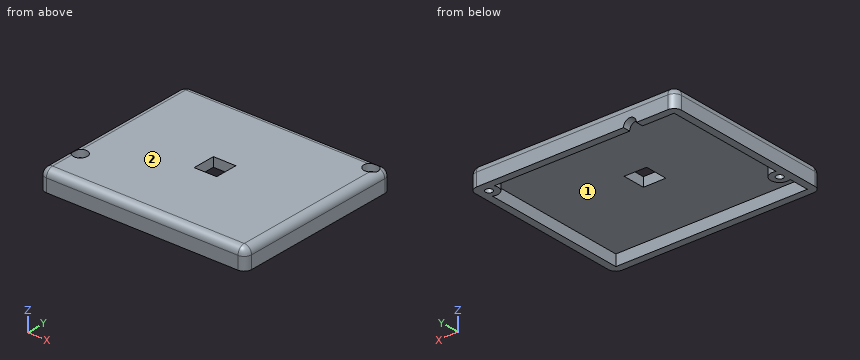
Autodesk Inventor part; units mm, degrees
ref_plane "Arbeitsebene1" through (26, 12.1004, 0) normal (0, 0, 1) x (1, 0, 0)
ref_plane "YZ Plane" through (0, 0, 0) normal (1, 0, 0) x (0, 1, 0)
ref_plane "XZ Plane" through (0, 0, 0) normal (0, 1, 0) x (-1, 0, 0)
ref_plane "Arbeitsebene1" through (26, 12.1004, 0) normal (0, 0, 1) x (1, 0, 0)
sketch "Skizze1" plane through (26, 12.1004, 0) normal (0, 0, 1) x (1, 0, 0)
  arc A0 (-54, -33.6004) -> (-52, -35.6004) centre (-52, -33.6004) ccw
  line L0 (-52, -35.6004) -> (0, -35.6004)
  arc A1 (0, -35.6004) -> (2, -33.6004) centre (0, -33.6004) ccw
  line L1 (2, -33.6004) -> (2, 9.3996)
  arc A2 (2, 9.3996) -> (0, 11.3996) centre (0, 9.3996) ccw
  line L2 (0, 11.3996) -> (-52, 11.3996)
  arc A3 (-52, 11.3996) -> (-54, 9.3996) centre (-52, 9.3996) ccw
  line L3 (-54, 9.3996) -> (-54, -33.6004)
  circle A4 centre (-0.95, 8.4496) radius 0.95
  circle A5 centre (-51.05, -25.8004) radius 0.95
  arc A6 (-24.2441, 3.8663) -> (-23.5, 4.8331) centre (-24.5, 4.8331) ccw
  line L4 (-23.5, 5.8996) -> (-23.5, 4.8331)
  line L5 (-24.5, 5.8996) -> (-23.5, 5.8996)
  line L6 (-24.5, 9.3996) -> (-24.5, 5.8996)
  line L7 (-24.5, 9.3996) -> (-7.5, 9.3996)
  line L8 (-7.5, 5.8996) -> (-7.5, 9.3996)
  line L9 (-8.5, 5.8996) -> (-7.5, 5.8996)
  line L10 (-8.5, 4.8996) -> (-8.5, 5.8996)
  arc A7 (-8.5, 4.8996) -> (-7.5, 3.8996) centre (-7.5, 4.8996) ccw
  line L11 (-7, 3.8996) -> (-7.5, 3.8996)
  arc A8 (-7, 3.8996) -> (-6, 4.8996) centre (-7, 4.8996) ccw
  line L12 (-6, 9.3996) -> (-6, 4.8996)
  line L13 (-6, 9.3996) -> (-4.3996, 9.3996)
  arc A9 (-3.3997, 8.4141) -> (-4.3996, 9.3996) centre (-4.3996, 8.3996) ccw
  arc A10 (-3.3997, 8.4141) -> (-0.9855, 5.9999) centre (-0.95, 8.4496) ccw
  arc A11 (0, 5) -> (-0.9855, 5.9999) centre (-1, 5) ccw
  line L14 (0, 5) -> (0, -25.7504)
  arc A12 (-0.5, -26.6164) -> (0, -25.7504) centre (-1, -25.7504) ccw
  arc A13 (-0.5, -26.6164) -> (-1, -27.4824) centre (0, -27.4824) ccw
  line L15 (-1, -28.7504) -> (-1, -27.4824)
  line L16 (0, -28.7504) -> (-1, -28.7504)
  line L17 (0, -28.7504) -> (0, -33.6004)
  line L18 (0, -33.6004) -> (-52, -33.6004)
  line L19 (-52, -33.6004) -> (-52, -28.7504)
  line L20 (-51, -28.7504) -> (-52, -28.7504)
  line L21 (-51, -28.6986) -> (-51, -28.7504)
  arc A14 (-50.5932, -28.2074) -> (-51, -28.6986) centre (-50.5, -28.6986) ccw
  arc A15 (-50.5932, -28.2074) -> (-51.0145, -23.3506) centre (-51.05, -25.8004) ccw
  arc A16 (-52, -22.3507) -> (-51.0145, -23.3506) centre (-51, -22.3507) ccw
  line L22 (-52, -22.3507) -> (-52, 2.2996)
  arc A17 (-51.5, 3.1657) -> (-52, 2.2996) centre (-51, 2.2996) ccw
  arc A18 (-51.5, 3.1657) -> (-51, 4.0317) centre (-52, 4.0317) ccw
  line L23 (-51, 5.2996) -> (-51, 4.0317)
  line L24 (-52, 5.2996) -> (-51, 5.2996)
  line L25 (-52, 5.2996) -> (-52, 9.3996)
  line L26 (-52, 9.3996) -> (-26, 9.3996)
  line L27 (-26, 5.2996) -> (-26, 9.3996)
  line L28 (-27, 5.2996) -> (-26, 5.2996)
  line L29 (-27, 4.2996) -> (-27, 5.2996)
  arc A19 (-27, 4.2996) -> (-26, 3.2996) centre (-26, 4.2996) ccw
  line L30 (-25.4165, 3.2996) -> (-26, 3.2996)
  arc A20 (-25.4165, 3.2996) -> (-24.7024, 3.5996) centre (-25.4165, 4.2996) ccw
  arc A21 (-24.2441, 3.8663) -> (-24.7024, 3.5996) centre (-23.9882, 2.8996) ccw
  point P0 (-26, -12.1004)
extrude "Extrusion1" add sketch "Skizze1" along normal blind 2.5 contours L3 A3 L2 A2 L1 A1 L0 A0 | A6 L4 L5 L6 L7 L8 L9 L10 A7 L11 A8 L12 L13 A9 A10 A11 L14 A12 A13 L15 L16 L17 L18 L19 L20 L21 A14 A15 A16 L22 A17 A18 L23 L24 L25 L26 L27 L28 L29 A19 L30 A20 A21
sketch "Skizze2" plane through (26, 12.1004, 2.5) normal (0, 0, 1) x (1, 0, 0)
  circle A0 centre (-0.95, 8.4496) radius 0.95
  circle A1 centre (-51.05, -25.8004) radius 0.95
  circle A2 centre (-51.05, -25.8004) radius 1.9
  circle A3 centre (-0.95, 8.4496) radius 1.9
  point P0 (-26, -12.1004)
  dimension "d2" = 3.8
  dimension "d3" = 3.8
extrude "Extrusion2" cut sketch "Skizze2" against normal blind 2
fillet "Rundung1" radius 1.99 8 edges at (27.4142, 22.9142, 2.5) (0, 23.5, 2.5) (-27.4142, 22.9142, 2.5) (-28, 0, 2.5) (-27.4142, -22.9142, 2.5) (0, -23.5, 2.5) (27.4142, -22.9142, 2.5) (28, 0, 2.5)
sketch "Skizze3" plane through (26, 12.1004, 2.5) normal (0, 0, 1) x (1, 0, 0)
  line L0 (-22.95, -9.0004) -> (-29.05, -9.0004)
  line L1 (-29.05, -9.0004) -> (-29.05, -15.2004)
  line L2 (-29.05, -15.2004) -> (-22.95, -15.2004)
  line L3 (-22.95, -15.2004) -> (-22.95, -9.0004)
  line L4 (-22.95, -9.0004) -> (-29.05, -15.2004) construction
  line L5 (-29.05, -9.0004) -> (-22.95, -15.2004) construction
  point P0 (-26, -12.1004)
  dimension "d7" = 6.1
  dimension "d8" = 6.2
extrude "Extrusion3" cut sketch "Skizze3" against normal through all
sketch "Skizze5" plane through (26, 12.1004, 0) normal (0, 0, -1) x (-1, 0, 0)
  line L0 (0, 9.3996) -> (52, 9.3996)
  line L1 (52, 9.3996) -> (52, -33.6004)
  line L2 (52, -33.6004) -> (0, -33.6004)
  line L3 (0, -33.6004) -> (0, 9.3996)
  line L4 (0, 11.3996) -> (52, 11.3996)
  line L5 (52, -35.6004) -> (0, -35.6004)
  line L6 (54, 9.3996) -> (54, -33.6004)
  line L7 (-2, -33.6004) -> (-2, 9.3996)
  line L8 (29.05, -15.2004) -> (22.95, -15.2004)
  line L9 (22.95, -15.2004) -> (22.95, -9.0004)
  line L10 (22.95, -9.0004) -> (29.05, -9.0004)
  line L11 (29.05, -9.0004) -> (29.05, -15.2004)
  line L12 (52, -35.6004) -> (0, -35.6004)
  arc A0 (52, -35.6004) -> (54, -33.6004) centre (52, -33.6004) ccw
  line L13 (54, 9.3996) -> (54, -33.6004)
  arc A1 (54, 9.3996) -> (52, 11.3996) centre (52, 9.3996) ccw
  line L14 (0, 11.3996) -> (52, 11.3996)
  arc A2 (0, 11.3996) -> (-2, 9.3996) centre (0, 9.3996) ccw
  line L15 (-2, -33.6004) -> (-2, 9.3996)
  arc A3 (-2, -33.6004) -> (0, -35.6004) centre (0, -33.6004) ccw
  circle A4 centre (0.95, 8.4496) radius 0.95
  circle A5 centre (51.05, -25.8004) radius 0.95
  point P0 (26, -12.1004)
  point P1 (54, -33.6004)
  point P2 (54, 9.3996)
  point P3 (52, 11.3996)
  point P4 (0, 11.3996)
  point P5 (-2, 9.3996)
  point P6 (-2, -33.6004)
  point P7 (0, -35.6004)
  dimension "d11" = 2
  dimension "d12" = 2
  dimension "d13" = 2
  dimension "d14" = 2
extrude "Extrusion4" add sketch "Skizze5" along normal blind 3 contours L4 A1 L6 A0 L5 A3 L7 A2
sketch "Skizze6" plane through (-26, 23.5, 0.51) normal (0, 1, 0) x (1, 0, 0)
  line L0 (52, 3.51) -> (0, 3.51)
  circle A0 centre (10.3315, 3.51) radius 1.75
  point P0 (26, 0.51)
  point P1 (8.5815, 3.51)
  point P2 (12.0815, 3.51)
  dimension "d17" = 3.5
extrude "Extrusion5" cut sketch "Skizze6" against normal blind 3 contours A0 L0 picked at (10.0001, 3.0299)
sketch "Skizze7" plane through (26, 12.1004, 0) normal (0, 0, -1) x (-1, 0, 0)
  line L0 (29.05, -15.2004) -> (22.95, -15.2004)
  line L1 (22.95, -15.2004) -> (22.95, -9.0004)
  line L2 (22.95, -9.0004) -> (29.05, -9.0004)
  line L3 (29.05, -9.0004) -> (29.05, -15.2004)
  line L4 (52, 9.3996) -> (0.95, 9.3996)
  arc A0 (0, 8.4496) -> (0.95, 9.3996) centre (0.95, 8.4496) ccw
  line L5 (0, 8.4496) -> (0, -33.6004)
  line L6 (0, -33.6004) -> (52, -33.6004)
  line L7 (52, -33.6004) -> (52, -25.8004)
  circle A1 centre (51.05, -25.8004) radius 0.95
  line L8 (52, -25.8004) -> (52, 9.3996)
  circle A2 centre (51.05, -25.8004) radius 2.45
  circle A3 centre (0.95, 8.4496) radius 2.45
  line L9 (39.9185, 9.3996) -> (39.9185, 11.3996)
  line L10 (39.9185, 11.3996) -> (0, 11.3996)
  arc A4 (0, 11.3996) -> (-2, 9.3996) centre (0, 9.3996) ccw
  line L11 (-2, 9.3996) -> (-2, -33.6004)
  arc A5 (-2, -33.6004) -> (0, -35.6004) centre (0, -33.6004) ccw
  line L12 (0, -35.6004) -> (52, -35.6004)
  arc A6 (52, -35.6004) -> (54, -33.6004) centre (52, -33.6004) ccw
  line L13 (54, -33.6004) -> (54, 9.3996)
  arc A7 (54, 9.3996) -> (52, 11.3996) centre (52, 9.3996) ccw
  line L14 (52, 11.3996) -> (43.4185, 11.3996)
  line L15 (43.4185, 11.3996) -> (43.4185, 9.3996)
  line L16 (43.4185, 9.3996) -> (52, 9.3996)
  line L17 (52, 9.3996) -> (52, -33.6004)
  line L18 (52, -33.6004) -> (0, -33.6004)
  line L19 (0, -33.6004) -> (0, 9.3996)
  line L20 (0, 9.3996) -> (39.9185, 9.3996)
  arc A8 (0.95, 9.3996) -> (0, 8.4496) centre (0.95, 8.4496) ccw
  point P0 (26, -12.1004)
  point P1 (52, -23.542)
  point P2 (52, -28.0587)
  point P3 (0.95, 9.3996)
  point P4 (0.95, 9.3996)
  point P5 (0.95, 9.3996)
  point P6 (3.2083, 9.3996)
  point P7 (0, 6.1913)
  dimension "d20" = 1.5
  dimension "d21" = 1.5
extrude "Extrusion6" add sketch "Skizze7" along normal blind 3 contours L8 L7 A2 | A3 L5 A0 L4 | A8 L19 L20 picked at (49.1338, -25.5256)
properties part number "Lid"
Could you check a few things on this model? Use its own coordinates, in mm. Face numbers are marked on the shaded views. Round coordinates to 2 decimals unless told otherwise and drop trailing zeros. Loops run counter-clockwise (first coordinate to the right, second up) from the corner with the lowest first, then second, coordinate; pieces in that order, holes last.
Q1. Thinking about a two-plate mould opening in Y: for the marked faces 1 and 2, which applies, pulls with the +Y half, pulls with the -Y half, needs draft (parallel to the pull), parting line crosses it, or undercut?
Q2. For P1, Ø1.2, axis at x = 0.5, z = 1.5, coming from the +Y side; P2, Ø1.2, axis at y = 1, z = 1.5, coming from the -X side; P3, Ø3, axis at x = 25.5, y = 21.5, coming from the +Z side, each with a flat end and sliding along its axis, tell me the tip position at first contact or that it passes through.
Q3. I want a section at D-D (z = -2.4). Write out the boundary of the cut face in (x, y), and give its area (3 significant figures).
Q4. Please list where these lines run through material, in increasing order: L1, parallel to Y at x = -25.05, z = -0.8; L2, parallel to Y at x = 25.05, z = -1.95; L3, parallel to Y at x = -16.5, z = -0.2.
Q5. I want a section at B-B (y = -2.5). Write out the boundary of the cut face in (x, z).
Q6. I want a section at A-A (x = -25.05). Write out the boundary of the cut face in (y, z), and give its area (3 significant figures).
Q7. I want a section at C-C (x = 8). Write out the boundary of the cut face in (y, z).
Answer below:
1. face 1: undercut
1. face 2: needs draft
2. P1: stops at y = 23.46
2. P2: stops at x = -27.96
2. P3: stops at z = 2.42
3. outline: (-28, -21.5) arc R2 ccw to (-26, -23.5) - (26, -23.5) arc R2 ccw to (28, -21.5) - (28, 21.5) arc R2 ccw to (26, 23.5) - (-14.02, 23.5) - (-14.02, 21.5) - (22.79, 21.5) arc R2.45 ccw to (26, 18.29) - (26, -21.5) - (-26, -21.5) - (-26, -15.96) arc R2.45 ccw (long way) to (-26, -11.44) - (-26, 21.5) - (-17.31, 21.5) - (-17.31, 23.5) - (-26, 23.5) arc R2 ccw to (-28, 21.5) - close; hole circle Ø1.9 at (-25.05, -13.7); hole circle Ø1.9 at (25.05, 20.55)
3. area: 404 mm2
4. L1: y = -23.5 to -21.5, -16.15 to -14.65, -12.75 to -11.25, 21.5 to 23.5
4. L2: y = -23.5 to -21.5, 18.1 to 19.6, 21.5 to 23.5
4. L3: y = -23.5 to -21.5, 21.5 to 23.5
5. outline: (-28, -3) - (-26, -3) - (-26, 0) - (-3.05, 0) - (-3.05, 2.5) - (-26.01, 2.5) arc R1.99 ccw to (-28, 0.51) - close; (3.05, 0) - (26, 0) - (26, -3) - (28, -3) - (28, 0.51) arc R1.99 ccw to (26.01, 2.5) - (3.05, 2.5) - close
6. outline: (-23.5, -3) - (-21.5, -3) - (-21.5, 0) - (-16.15, 0) - (-16.15, -3) - (-14.65, -3) - (-14.65, 0.5) - (-15.6, 0.5) - (-15.6, 2.5) - (-21.51, 2.5) arc R1.99 ccw to (-23.5, 0.51) - close; (-12.75, -3) - (-11.25, -3) - (-11.25, 0) - (21.5, 0) - (21.5, -3) - (23.5, -3) - (23.5, 0.51) arc R1.99 ccw to (21.51, 2.5) - (-11.8, 2.5) - (-11.8, 0.5) - (-12.75, 0.5) - close
6. area: 128 mm2
7. outline: (-23.5, -3) - (-21.5, -3) - (-21.5, 0) - (21.5, 0) - (21.5, -3) - (23.5, -3) - (23.5, 0.51) arc R1.99 ccw to (21.51, 2.5) - (-21.51, 2.5) arc R1.99 ccw to (-23.5, 0.51) - close
